Part model, mm, in its own coordinate system. A direction names the side the tool comes from. Coordinates: 2 decimals unless noted, no trailing zeros. Loops run counter-clockwise (first coordinate to the right, second up) from the corner with the lowest first, then second, coordinate; pieces in that order, holes last. Notation, with made-up numbers: (48.25, -4) - (103.25, -4) arc R19 cw to (103.25, 10) - close; hole circle Ø9 at (34, 3). An arc over 180 degrees is marked (long way). Use a Markdown table: item, result. Add a question column.
1. Band-saw the part on B-B, the plane x = -33. Give the cut face in (y, z) (3 decimals).
2. Band-saw the part on C-C, the plane x = -6. Give the cut face in (y, z) (3 decimals), plus the area to 3 significant figures.
3. Band-saw the part on A-A, the plane y = 0.7. Give the cut face in (x, z), plus the area to 3 significant figures.
4. Wall check: probe 1 along Z at (x, y) = (0.5, 2.5); probe 2 along X at (y, z) = (1.95, -150.5); probe 3 along Z at (x, y) = (29.5, 1.05). Give the ranges that are in metal, low to high. Write a range as [from, to].
5. 3-axis set-ups, long thin cutter, end or side, ignore diameter. For faces 1 (the cylindrical face through (-61.084, 1.61, -163.466)), 2 (the flat face through (-1, 0, -2)): which of +Z, -Z, +X, -X, +Y, -Y reach the whole face in a straight line?
from build123d import *

# Parameters (mm, degrees)
SKETCH1_W           = 203.2
SKETCH1_H           = 342.9
BOSS_EXTRUDE1_DEPTH = 3.175
CUT_EXTRUDE1_DEPTH  = 200.31819567
FILLET1_R           = 127


with BuildPart() as part:
    # Sketch1 → Boss-Extrude1 (new body)
    with BuildSketch(Plane(origin=(0, 0, 0), x_dir=(1, 0, 0), z_dir=(0, 1, 0))):
        Rectangle(SKETCH1_W, SKETCH1_H)
    extrude(amount=BOSS_EXTRUDE1_DEPTH)

    # Sketch2 → Cut-Extrude1 (cut, through all)
    with BuildSketch(Plane(origin=(0, 3.175, 0), x_dir=(1, 0, 0), z_dir=(0, 1, 0))):
        with BuildLine():
            ThreePointArc((-38.1, 171.45), (0, 133.35), (38.1, 171.45))
            Line((38.1, 171.45), (-38.1, 171.45))
        make_face()
    extrude(amount=-CUT_EXTRUDE1_DEPTH, mode=Mode.SUBTRACT)

    # Fillet1
    # the kernel refuses this fillet: 127 mm, written as the material it takes off along each edge
    with BuildSketch(Plane(origin=(38.1, 161.925, -171.45), x_dir=(-0.42460388780422365, 0, 0.905379223564103), z_dir=(0, -1, 0))) as fillet1_piece_1:
        with BuildLine():
            CenterArc((86.279510002, -114.983161393), FILLET1_R, 115.12559338, 37.958028581)
            Line((-26.962346876, -57.491580696), (-29.227184013, -56.341749082))
            ThreePointArc((-29.227184013, -56.341749082), (-15.780836666, -27.667296473), (-2.299663228, 1.078493875))
            Line((-2.299663228, 1.078493875), (1.078493875, 2.299663228))
            ThreePointArc((1.078493875, 2.299663228), (16.177408125, -1.065051582), (31.276322376, 2.299663228))
            Line((31.276322376, 2.299663228), (32.354816251, 0))
        make_face()
    extrude(amount=320.675, mode=Mode.SUBTRACT)
    with BuildSketch(Plane(origin=(-38.1, 161.925, -171.45), x_dir=(-1, 0, 0), z_dir=(0, -1, 0))) as fillet1_piece_2:
        with BuildLine():
            CenterArc((67.46875, -126.937973134), FILLET1_R, 91.790784659, 37.958028581)
            Line((-13.737980769, -29.293378416), (-15.362115385, -27.340486521))
            ThreePointArc((-15.362115385, -27.340486521), (-5.90471481, -15.09891425), (-2.54, 0))
            Line((-2.54, 0), (0, 2.54))
            ThreePointArc((0, 2.54), (31.75, 2.54), (63.420625, 2.538759463))
            Line((63.420625, 2.538759463), (63.5, 0))
        make_face()
    extrude(amount=320.675, mode=Mode.SUBTRACT)


solid = part.part
Geometry check:
| question | item | result |
|---|---|---|
| 1 | outline | (0, -148.737) - (3.175, -148.737) - (3.175, 171.45) - (0, 171.45) - close |
| 2 | outline | (0, -133.825) - (3.175, -133.825) - (3.175, 171.45) - (0, 171.45) - close |
| 2 | area | 969 mm^2 |
| 3 | outline | (-101.6, -171.45) arc R127 ccw to (-24.36, -142.16) arc R38.1 cw to (24.36, -142.16) arc R127 ccw to (101.6, -171.45) - (101.6, 171.45) - (-101.6, 171.45) - close |
| 3 | area | 66,500 mm^2 |
| 4 | probe 1 | z = [-133.35, 171.45] |
| 4 | probe 2 | x = [-101.6, -35.6], [35.6, 101.6] |
| 4 | probe 3 | z = [-146.21, 171.45] |
| 5 | face 1 | -Z, +Y, -Y |
| 5 | face 2 | +Z, -Z, +X, -X, -Y |
